from build123d import *

# Parameters (mm, degrees)
SKETCH_1_W      = 45
SKETCH_1_H      = 75
SKETCH_1_R      = 2
SKETCH_1_R_2    = 1.5
SKETCH_1_R_3    = 3.5
EXTRUDE_1_DEPTH = 3
FILLET_1_R      = 6


with BuildPart() as part:
    # 草图1 → 凸台-拉伸1 (new body)
    with BuildSketch(Plane.XY):
        Rectangle(SKETCH_1_W, SKETCH_1_H)
        with Locations((-15, 10.5)):
            Circle(SKETCH_1_R, mode=Mode.SUBTRACT)
        with Locations((15, 10.5)):
            Circle(SKETCH_1_R, mode=Mode.SUBTRACT)
        with Locations((15, -31.5)):
            Circle(SKETCH_1_R, mode=Mode.SUBTRACT)
        with Locations((-15, -31.5)):
            Circle(SKETCH_1_R, mode=Mode.SUBTRACT)
        with Locations((0, 32.5)):
            Circle(SKETCH_1_R_2, mode=Mode.SUBTRACT)
        with Locations((7, 25.5)):
            Circle(SKETCH_1_R_2, mode=Mode.SUBTRACT)
        with Locations((0, 18.5)):
            Circle(SKETCH_1_R_2, mode=Mode.SUBTRACT)
        with Locations((-7, 25.5)):
            Circle(SKETCH_1_R_2, mode=Mode.SUBTRACT)
        with Locations((0, 25.5)):
            Circle(SKETCH_1_R_3, mode=Mode.SUBTRACT)
    extrude(amount=EXTRUDE_1_DEPTH)

    # 圆角1
    fillet_1_edges = [part.edges().sort_by_distance(p)[0] for p in [
        (22.5, -37.5, 1.5),
        (-22.5, -37.5, 1.5),
        (-22.5, 37.5, 1.5),
        (22.5, 37.5, 1.5),
    ]]
    fillet(fillet_1_edges, radius=FILLET_1_R)


solid = part.part
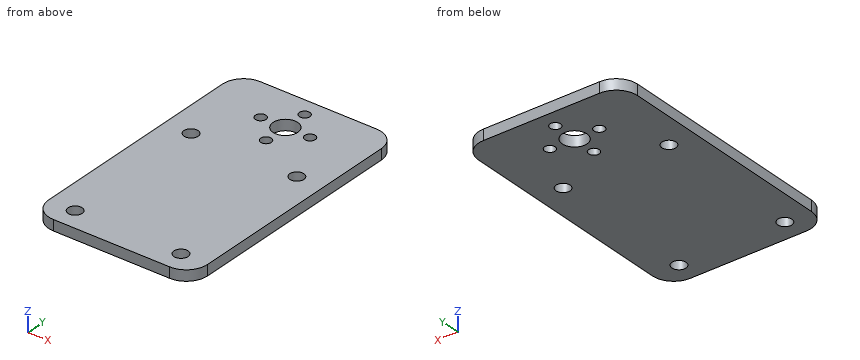
Build history of the part. All positions in model axes, mm. Round coordinates to 2 decimals unless told otherwise and drop trailing zeros. Write each loop counter-clockwise with the first axis right and the second up, starting at its lowest first coordinate (ties: lowest second). Pieces come first, ordered by that corner, then holes. Notation, with made-up numbers: M 84,-22 L 126,-22 A16 ccw 126,-18 Z; hole C 88,73.5 d11. An arc over 180 degrees is marked long. Answer in a Markdown table with one row per item.
1. Saw through at D-D (x = -7). List the corners of the cut face in (y, z), and give its area (3 significant figures).
Geometry check:
| item | result |
|---|---|
| outline | M -37.5,0 L 24,0 L 24,3 L -37.5,3 Z; M 27,0 L 37.5,0 L 37.5,3 L 27,3 Z |
| area | 216 mm2 |
2. Flat gauge pin, fed straight in: P1, Ø3, axis at x = -15, y = -31.5, coming from the +Z side. Where does the tip first touch, or does it go through?
Geometry check:
| item | result |
|---|---|
| P1 | through |
3. Saw through at C-C (x = 0). List the corners of the cut face in (y, z).
Geometry check:
| item | result |
|---|---|
| outline | M -37.5,0 L 17,0 L 17,3 L -37.5,3 Z; M 20,0 L 22,0 L 22,3 L 20,3 Z; M 29,0 L 31,0 L 31,3 L 29,3 Z; M 34,0 L 37.5,0 L 37.5,3 L 34,3 Z |
4. Saw through at A-A (y = 25.5). List the corners of the cut face in (x, z).
Geometry check:
| item | result |
|---|---|
| outline | M -22.5,0 L -8.5,0 L -8.5,3 L -22.5,3 Z; M -5.5,0 L -3.5,0 L -3.5,3 L -5.5,3 Z; M 3.5,0 L 5.5,0 L 5.5,3 L 3.5,3 Z; M 8.5,0 L 22.5,0 L 22.5,3 L 8.5,3 Z |
5. Probe L1, parallel to Y at x = -15, z = 1.3; L2, parallel to Y at x = 0, z = 1.45; L3, parallel to Y at x = 13.5, z = 1.8. List the from-to ranges inside material, lowest first. Write a range as [from, to].
Geometry check:
| item | result |
|---|---|
| L1 | [-37.5, -33.5], [-29.5, 8.5], [12.5, 37.5] |
| L2 | [-37.5, 17], [20, 22], [29, 31], [34, 37.5] |
| L3 | [-37.5, -32.82], [-30.18, 9.18], [11.82, 37.5] |
6. Saw through at B-B (x = -15). List the corners of the cut face in (y, z), and give its area (3 significant figures).
Geometry check:
| item | result |
|---|---|
| outline | M -37.5,0 L -33.5,0 L -33.5,3 L -37.5,3 Z; M -29.5,0 L 8.5,0 L 8.5,3 L -29.5,3 Z; M 12.5,0 L 37.5,0 L 37.5,3 L 12.5,3 Z |
| area | 201 mm2 |
